Can you work these out from the drawing? Everything is in mm from the part's minimum corner. Give positions to 0.01 mm unless a question says otherwise; leave off trailing zeros. Write each loop counter-clockwise with the first axis right and the second up, starting at its lowest first coordinate (ties: lowest second). Pieces come first, ordered by that corner, then holes. Notation, with made-up numbers: M -0.75,47 L 19.25,47 A5 cw 19.25,54 Z; hole C 80,81.5 d3. An arc over 180 degrees is marked long. One line per item, written item: value.
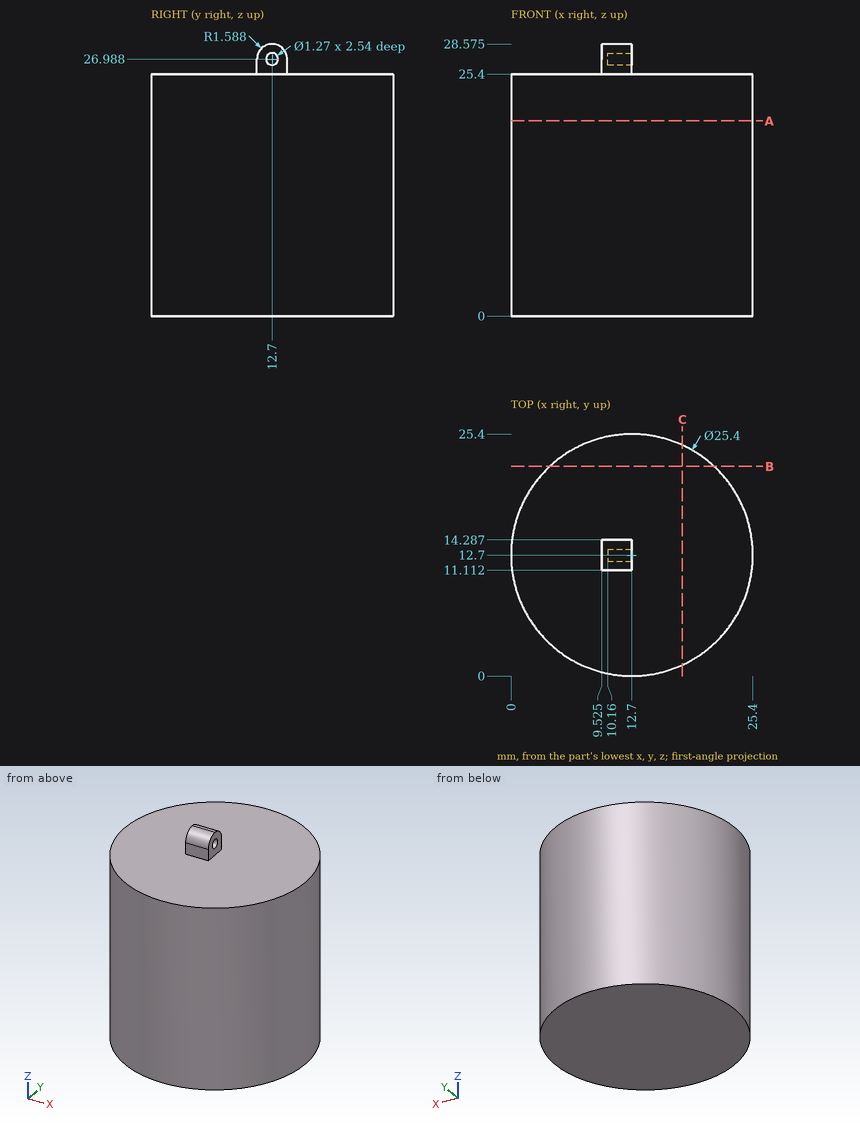
1) If we section it at B-B, the plane y = 22: Write out the boundary of the cut face in (x, z).
Outcome:
outline: M 4.05,0 L 21.35,0 L 21.35,25.4 L 4.05,25.4 Z
2) I'm going to push flat-ended pins straight in: pin 1 (1 mm diameter, centred on x = 11, z = 17.5, fed in from -Y); pin 2 (8 mm diameter, centred on x = 9.5, y = 8, fed in from -Z); pin 3 (2 mm diameter, centred on y = 12.7, z = 26.99, fed in from -X) (1 decimal); pin 4 (0.5 mm diameter, centred on x = 12, z = 26, fed in from -Y). Where does each tip first touch, or does it pass through?
Outcome:
pin 1: stops at y = 0.06
pin 2: stops at z = 0
pin 3: stops at x = 9.5
pin 4: stops at y = 11.11
3) If we section it at A-A, the plane z = 20.5: Write out the boundary of the cut face in (x, y), then the cut area to 3 significant figures.
Outcome:
outline: C 12.7,12.7 d25.4
area: 507 mm^2
4) Please list where these lines run through material, in increasing order: L1, parallel to Z at x = 8.75, y = 15.5; L2, parallel to Y at x = 11.5, z = 26; L3, parallel to X at y = 8, z = 20. Write a range as from..to.
Outcome:
L1: z = 0..25.4
L2: y = 11.11..14.29
L3: x = 0.9..24.5
5) If we section it at C-C, the plane x = 18: Write out the boundary of the cut face in (y, z).
Outcome:
outline: M 1.16,0 L 24.24,0 L 24.24,25.4 L 1.16,25.4 Z
